```python
from build123d import *

# Parameters (mm, degrees)
BOSS_EXTRUDE1_DEPTH = 15.8
SKETCH2_R           = 2
CUT_EXTRUDE1_DEPTH  = 15.8
SKETCH4_R           = 2
CUT_EXTRUDE2_DEPTH  = 15.8
SKETCH5_R           = 1.5
CUT_EXTRUDE3_DEPTH  = 34.624990706


with BuildPart() as part:
    # Sketch1 → Boss-Extrude1 (new body)
    with BuildSketch(Plane.XY):
        with BuildLine():
            Line((0, 0), (34, 0))
            Line((34, 0), (34, 3))
            Line((34, 3), (25, 3))
            Line((25, 3), (25, 16))
            Line((25, 16), (17.5, 16))
            Line((17.5, 16), (17.5, 11))
            ThreePointArc((17.5, 11), (17, 3.031373033), (16.5, 11))
            Line((16.5, 11), (16.5, 16))
            Line((16.5, 16), (9, 16))
            Line((9, 16), (9, 3))
            Line((9, 3), (0, 3))
            Line((0, 3), (0, 0))
        make_face()
    extrude(amount=-BOSS_EXTRUDE1_DEPTH)

    # Sketch2 → Cut-Extrude1 (cut)
    with BuildSketch(Plane(origin=(0, 3, 0), x_dir=(1, 0, 0), z_dir=(0, 1, 0))):
        with Locations(Location((4.5, 7.9, 0), (0, 0, 270))):
            Circle(SKETCH2_R)
    extrude(amount=-CUT_EXTRUDE1_DEPTH, mode=Mode.SUBTRACT)

    # Sketch4 → Cut-Extrude2 (cut)
    with BuildSketch(Plane(origin=(0, 3, 0), x_dir=(1, 0, 0), z_dir=(0, 1, 0))):
        with Locations(Location((29.5, 7.9, 0), (0, 0, 270))):
            Circle(SKETCH4_R)
    extrude(amount=-CUT_EXTRUDE2_DEPTH, mode=Mode.SUBTRACT)

    # Sketch5 → Cut-Extrude3 (cut, through all)
    with BuildSketch(Plane(origin=(25, 0, 0), x_dir=(0, 0, -1), z_dir=(1, 0, 0))):
        with Locations((7.9, 13.5)):
            Circle(SKETCH5_R)
    extrude(amount=-CUT_EXTRUDE3_DEPTH, mode=Mode.SUBTRACT)


solid = part.part
```
Build history of the part. All positions in model axes, mm. A direction names the side the tool comes from. Give positions to 0.01 mm unless a question says otherwise; leave off trailing zeros. Loops run counter-clockwise (first coordinate to the right, second up) from the corner with the lowest first, then second, coordinate; pieces in that order, holes last.
1) Band-saw the part on B-B on y = 13.5. List the corners of the cut face in (x, z).
Values follow:
outline: (9, -15.8) - (16.5, -15.8) - (16.5, -9.4) - (9, -9.4) - close; (9, -6.4) - (16.5, -6.4) - (16.5, 0) - (9, 0) - close; (17.5, -15.8) - (25, -15.8) - (25, -9.4) - (17.5, -9.4) - close; (17.5, -6.4) - (25, -6.4) - (25, 0) - (17.5, 0) - close
2) Two-plate mould, pull along Z, no slides. Class faces 1 (the face through (21.3, 12.6, -6.7)), 2 (the face through (17.169, 3.035, -7.789)), 3 (the face through (12.98, 8.11, 0)): released by +Z, released by -Z, zero draft, split by the parting line, or undercut.
Values follow:
face 1: undercut
face 2: zero draft
face 3: released by +Z
3) 3-axis set-ups, long thin cutter, end or side, ignore diameter. For faces 4 (the face through (9, 10, -8)), 5 (the face through (16.5, 11.8, -7.8)), 6 (the face through (12.8, 12.6, -6.7)), 7 (the face through (31, 3, -6)): which of +Z, -Z, +X, -X, +Y, -Y reach the whole face in a straight line?
Values follow:
face 4: +Z, -Z, -X, +Y
face 5: +Z, -Z, +Y
face 6: +X, -X
face 7: +Z, -Z, +X, +Y
4) Band-saw the part on A-A on x = 18. List the corners of the cut face in (y, z), then the cut area to 3 significant figures.
Values follow:
outline: (0, -15.8) - (3.16, -15.8) - (3.16, 0) - (0, 0) - close; (10.9, -15.8) - (16, -15.8) - (16, 0) - (10.9, 0) - close; hole circle Ø3 at (13.5, -7.9)
area: 123 mm2
5) Band-saw the part on C-C on z = -7.9. List the corners of the cut face in (x, y), then the cut area to 3 significant figures.
Values follow:
outline: (0, 0) - (2.5, 0) - (2.5, 3) - (0, 3) - close; (6.5, 0) - (27.5, 0) - (27.5, 3) - (25, 3) - (25, 12) - (17.5, 12) - (17.5, 11) arc R4 cw (long way) to (16.5, 11) - (16.5, 12) - (9, 12) - (9, 3) - (6.5, 3) - close; (9, 15) - (16.5, 15) - (16.5, 16) - (9, 16) - close; (17.5, 15) - (25, 15) - (25, 16) - (17.5, 16) - close; (31.5, 0) - (34, 0) - (34, 3) - (31.5, 3) - close
area: 186 mm2
6) Probe line 1 along X through (y, z) = (0.8, -7.9); line 2 along X through (y, z) = (14.5, -3.5); line 3 along X through (y, z) = (7, -12.5). List the from-to ranges inside material, lowest first.
Values follow:
line 1: x = 0 to 2.5, 6.5 to 27.5, 31.5 to 34
line 2: x = 9 to 16.5, 17.5 to 25
line 3: x = 9 to 13, 21 to 25
7) Drop flat-ended pins along their axis: P1, Ø4, axis at y = 9, z = -10, coming from the +X side; P2, Ø4.5, axis at x = 2.5, z = -8.5, coming from the +Y side; P3, Ø1.5, axis at y = 10, z = -6, coming from the -X side. Give the stop position or say it passes through.
Values follow:
P1: stops at x = 25
P2: stops at y = 3
P3: stops at x = 9
8) Band-saw the part on D-D on x = 4.5. List the corners of the cut face in (y, z).
Values follow:
outline: (0, -15.8) - (3, -15.8) - (3, -9.9) - (0, -9.9) - close; (0, -5.9) - (3, -5.9) - (3, 0) - (0, 0) - close
